from build123d import *

# Parameters (mm, degrees)
F1_DEPTH = 468
F2_ANGLE = 180
F3_ANGLE = 90


with BuildPart() as f1:
    # F0 (on Front) → F1 (new body, symmetric)
    with BuildSketch(Plane.XZ):
        Polygon((-19.4449553564, 13.8652742597), (-21.0449553564, 13.8951456954), (-21.0449553564, -1.1048543046), (-6.0449553564, -1.1048543046), (-6.0449553564, 0.4951456954), (-19.4449553564, 0.4951456954), align=None)
    extrude(amount=F1_DEPTH, both=True)


with BuildPart() as f1_1:
    # F2: moved
    add(f1.part.rotate(Axis((-21.0449553564, 0, -1.1048543046), (0, -1, 0)), F2_ANGLE))


with BuildPart() as f1_2:
    # F3: moved
    add(f1_1.part.rotate(Axis((-21.0449553564, -468, -8.6048543046), (0, 0, 1)), F3_ANGLE))


solid = f1_2.part
Read the model definition and answer for the solid it produces. Units are mm, in the model's axes. Coordinates: 2 decimals unless noted, no trailing zeros. Loops run counter-clockwise (first coordinate to the right, second up) from the corner with the lowest first, then second, coordinate; pieces in that order, holes last.
Q1. The part is cut by section A-A on x = -838.5. Write down the section's boundary in (y, z), and give its area (3 significant figures).
Q2. The part is cut by section B-B on z = -13. Write down the section's boundary in (x, y), and give its area (3 significant figures).
Q3. Consider probe 1 along Y at (x, z) = (-462.5, -12.25); probe 2 along Z at (x, y) = (-318, -482); probe 3 along Z at (x, y) = (-793, -469). Determine where each line is inside the solid, lowest interval first.
Q4. The part is cut by section C-C on y = -473.5. Write down the section's boundary in (x, z).
Q5. Each of these flat-tipped pins is pushed along its axis until it touches: pin 1 Ø1 at (y, z) = (-471.5, -6.5) entering from -X; pin 2 Ø6.5 at (x, z) = (-503.5, -12) entering from -Y; pin 3 Ø1.5 at (x, y) = (-360, -480.5) entering from -Z. Where does it stop, or does it pass through?
Results below:
1. outline: (-483, -2.7) - (-469.6, -2.7) - (-469.6, -16.07) - (-468, -16.1) - (-468, -1.1) - (-483, -1.1) - close
1. area: 45.4 mm2
2. outline: (-957.04, -469.6) - (-21.04, -469.6) - (-21.04, -468) - (-957.04, -468) - close
2. area: 1,500 mm2
3. probe 1: y = -469.6 to -468
3. probe 2: z = -2.7 to -1.1
3. probe 3: z = -16.09 to -1.1
4. outline: (-957.04, -2.7) - (-21.04, -2.7) - (-21.04, -1.1) - (-957.04, -1.1) - close
5. pin 1: passes through
5. pin 2: stops at y = -469.6
5. pin 3: stops at z = -2.7
